Input: part model. Units: mm. Frame: model coordinates. A direction names the side the tool comes from. Give positions to 0.01 mm unless a question says otherwise; leave off trailing zeros. Loops run counter-clockwise (first coordinate to the right, second up) from the corner with the lowest first, then second, coordinate; pieces in that order, holes last.
from build123d import *

# Parameters (mm, degrees)
SKETCH1_W           = 156.4
SKETCH1_H           = 55
BOSS_EXTRUDE1_DEPTH = 3.175
SKETCH2_R           = 1.524
CUT_EXTRUDE1_DEPTH  = 83.955232656
SKETCH4_R           = 1.6
CUT_EXTRUDE2_DEPTH  = 83.955232656
SKETCH5_W           = 20
SKETCH5_H           = 20
CUT_EXTRUDE3_DEPTH  = 83.955232656
FILLET1_R           = 5


with BuildPart() as part:
    # Sketch1 → Boss-Extrude1 (new body)
    with BuildSketch(Plane(origin=(0, 0, 0), x_dir=(1, 0, 0), z_dir=(0, 1, 0))):
        Rectangle(SKETCH1_W, SKETCH1_H)
    extrude(amount=BOSS_EXTRUDE1_DEPTH)

    # Sketch2 → Cut-Extrude1 (cut, through all)
    with BuildSketch(Plane(origin=(0, 3.175, 0), x_dir=(1, 0, 0), z_dir=(0, 1, 0))):
        with Locations(Location((-68.547999997, -10.795000003, 0), (0, 0, 270))):
            Circle(SKETCH2_R)
        with Locations(Location((-62.197999997, -10.795000003, 0), (0, 0, 270))):
            Circle(SKETCH2_R)
        with Locations(Location((-55.847999997, -10.795000003, 0), (0, 0, 270))):
            Circle(SKETCH2_R)
        with Locations(Location((-49.497999997, -10.795000003, 0), (0, 0, 270))):
            Circle(SKETCH2_R)
        with Locations(Location((-43.147999997, -10.795000003, 0), (0, 0, 270))):
            Circle(SKETCH2_R)
        with Locations(Location((-36.797999997, -10.795000003, 0), (0, 0, 270))):
            Circle(SKETCH2_R)
        with Locations(Location((-68.547999997, 10.795000003, 0), (0, 0, 90))):
            Circle(SKETCH2_R)
        with Locations(Location((-62.197999997, 10.795000003, 0), (0, 0, 90))):
            Circle(SKETCH2_R)
        with Locations(Location((-55.847999997, 10.795000003, 0), (0, 0, 90))):
            Circle(SKETCH2_R)
        with Locations(Location((-49.497999997, 10.795000003, 0), (0, 0, 90))):
            Circle(SKETCH2_R)
        with Locations(Location((-43.147999997, 10.795000003, 0), (0, 0, 90))):
            Circle(SKETCH2_R)
        with Locations(Location((-36.797999997, 10.795000003, 0), (0, 0, 90))):
            Circle(SKETCH2_R)
        with Locations(Location((36.797999997, 10.795000003, 0), (0, 0, 270))):
            Circle(SKETCH2_R)
        with Locations(Location((43.147999997, 10.795000003, 0), (0, 0, 270))):
            Circle(SKETCH2_R)
        with Locations(Location((49.497999997, 10.795000003, 0), (0, 0, 270))):
            Circle(SKETCH2_R)
        with Locations(Location((55.847999997, 10.795000003, 0), (0, 0, 270))):
            Circle(SKETCH2_R)
        with Locations(Location((62.197999997, 10.795000003, 0), (0, 0, 270))):
            Circle(SKETCH2_R)
        with Locations(Location((68.547999997, 10.795000003, 0), (0, 0, 270))):
            Circle(SKETCH2_R)
        with Locations(Location((68.547999997, -10.795000003, 0), (0, 0, 90))):
            Circle(SKETCH2_R)
        with Locations(Location((62.197999997, -10.795000003, 0), (0, 0, 90))):
            Circle(SKETCH2_R)
        with Locations(Location((55.847999997, -10.795000003, 0), (0, 0, 90))):
            Circle(SKETCH2_R)
        with Locations(Location((49.497999997, -10.795000003, 0), (0, 0, 90))):
            Circle(SKETCH2_R)
        with Locations(Location((43.147999997, -10.795000003, 0), (0, 0, 90))):
            Circle(SKETCH2_R)
        with Locations(Location((36.797999997, -10.795000003, 0), (0, 0, 90))):
            Circle(SKETCH2_R)
    extrude(amount=-CUT_EXTRUDE1_DEPTH, mode=Mode.SUBTRACT)

    # Sketch4 → Cut-Extrude2 (cut, through all)
    with BuildSketch(Plane(origin=(0, 3.175, 0), x_dir=(1, 0, 0), z_dir=(0, 1, 0))):
        with Locations(Location((-67.2, -20.5, 0), (0, 0, 270))):
            Circle(SKETCH4_R)
        with Locations(Location((-67.2, 20.5, 0), (0, 0, 90))):
            Circle(SKETCH4_R)
        with Locations(Location((67.2, 20.5, 0), (0, 0, 270))):
            Circle(SKETCH4_R)
        with Locations(Location((67.2, -20.5, 0), (0, 0, 90))):
            Circle(SKETCH4_R)
    extrude(amount=-CUT_EXTRUDE2_DEPTH, mode=Mode.SUBTRACT)

    # Sketch5 → Cut-Extrude3 (cut, through all)
    with BuildSketch(Plane(origin=(0, 3.175, 0), x_dir=(1, 0, 0), z_dir=(0, 1, 0))):
        Rectangle(SKETCH5_W, SKETCH5_H)
    extrude(amount=-CUT_EXTRUDE3_DEPTH, mode=Mode.SUBTRACT)

    # Fillet1
    fillet1_edges = [part.edges().sort_by_distance(p)[0] for p in [
        (78.2, 1.5875, 27.5),
        (-78.2, 1.5875, 27.5),
        (-78.2, 1.5875, -27.5),
        (78.2, 1.5875, -27.5),
    ]]
    fillet(fillet1_edges, radius=FILLET1_R)


solid = part.part
(1) Cut plane C-C (y = 0.9). Count the separate pieces of the cut face and the enclosed holes in it, and give its area (3 significant figures).
Values follow:
separate pieces: 1
enclosed holes: 29
area: 7,970 mm2
(2) Reachability of faces 1 (the flat face through (-10, 2, 0)), 2 (the cylindrical face through (-76.77, 1.61, -26)) from +Z, -Z, +X, -X, +Y, -Y: full face, straight path, thin tool, end or side. Return the list, or none.
Values follow:
face 1: +Y, -Y
face 2: -Z, -X, +Y, -Y
(3) Cut plane A-A (z = 20.5). Return the cut outline in (x, y) (3 decimals), and give its area (3 significant figures).
Values follow:
outline: (-78.2, 0) - (-68.8, 0) - (-68.8, 3.175) - (-78.2, 3.175) - close; (-65.6, 0) - (65.6, 0) - (65.6, 3.175) - (-65.6, 3.175) - close; (68.8, 0) - (78.2, 0) - (78.2, 3.175) - (68.8, 3.175) - close
area: 476 mm2
(4) Mould query, pull axis X, two halves, no side actions, for faces 3 (the flat face through (78.2, 2, 0)), 4 (the cylindrical face through (-70.06, 1.61, -10.6)), 5 (the flat face through (-1, 3.175, -13)). Classes: +X half, -X half, draft (parallel to the pull), parting line (faces both ways), or undercut.
Values follow:
face 3: +X half
face 4: undercut
face 5: draft
(5) Ray query, probe 1 along X at (y, z) = (0.5, 20.5); probe 2 along X at (y, z) = (1.15, -21); probe 3 along Z at (x, y) = (66, 0.7). Return the intervals inside material, ascending.
Values follow:
probe 1: x = -78.2 to -68.8, -65.6 to 65.6, 68.8 to 78.2
probe 2: x = -78.2 to -68.72, -65.68 to 65.68, 68.72 to 78.2
probe 3: z = -27.5 to -21.56, -19.44 to 19.44, 21.56 to 27.5
(6) Cut plane B-B (z = 7). Return the cut outline in (x, y) (3 decimals).
Values follow:
outline: (-78.2, 0) - (-10, 0) - (-10, 3.175) - (-78.2, 3.175) - close; (10, 0) - (78.2, 0) - (78.2, 3.175) - (10, 3.175) - close
